Could you check a few things on this model? Use its own coordinates, in mm. A direction names the side the tool comes from. Give positions to 0.01 mm unless a question says otherwise; leave off trailing zeros. Order: outer loops, then holes, each group sorted by start corner. A loop starts at its lowest first (then second) coordinate and runs counter-clockwise, first axis right, second up. Notation, with made-up numbers: M -6.5,9 L 1.5,9 A18 ccw 1.5,26 Z; hole C 86.5,18.25 d3. An arc over 180 degrees is marked long. Use a Markdown table: item, result. Add a question column.
```python
from build123d import *

# Parameters (mm, degrees)
SKETCH_1_W                    = 520
SKETCH_1_H                    = 700
EXTRUDE_1_DEPTH               = 40
SKETCH_2_R                    = 23.1
CUT_EXTRUDE_1_DEPTH           = 873.926113712
CHAMFER_1_SIZE                = 4
M6X1_0_1_D                    = 5
CUT_EXTRUDE_2_DEPTH           = 873.926113712
HOLE_WIZARD_M10_1_D           = 10.5
HOLE_WIZARD_M10_1_CBORE_D     = 21.48
HOLE_WIZARD_M10_1_CBORE_DEPTH = 6.63
HOLE_WIZARD_M6_1_D            = 5
HOLE_WIZARD_M6_1_DEPTH        = 15
HOLE_WIZARD_M6_1_TIP          = 1.502151548


with BuildPart() as part:
    # 草图1 → 凸台-拉伸1 (new body)
    with BuildSketch(Plane.XY):
        with Locations((260, 350)):
            Rectangle(SKETCH_1_W, SKETCH_1_H)
    extrude(amount=EXTRUDE_1_DEPTH)

    # 草图2 → 切除-拉伸1 (cut, through all)
    with BuildSketch(Plane.XY.offset(40)):
        with Locations((140, 60)):
            Circle(SKETCH_2_R)
        with Locations((440, 60)):
            Circle(SKETCH_2_R)
        with Locations((440, 640)):
            Circle(SKETCH_2_R)
        with Locations((140, 640)):
            Circle(SKETCH_2_R)
    extrude(amount=-CUT_EXTRUDE_1_DEPTH, mode=Mode.SUBTRACT)

    # 倒角1
    chamfer_1_edges = [part.edges().sort_by_distance(p)[0] for p in [
        (520, 350, 40),
        (260, 700, 40),
        (0, 350, 40),
        (260, 700, 0),
        (520, 350, 0),
        (260, 0, 0),
        (0, 350, 0),
        (260, 0, 40),
        (0, 700, 20),
        (520, 700, 20),
        (520, 0, 20),
        (0, 0, 20),
    ]]
    chamfer(chamfer_1_edges, length=CHAMFER_1_SIZE)

    # M6x1.0 螺纹孔1 (through all)
    with Locations(Plane.XY.offset(40)):
        with Locations((25, 507.5), (150, 507.5), (275, 507.5), (275, 192.5), (150, 192.5), (25, 192.5)):
            Hole(M6X1_0_1_D / 2)

    # 草图5 → 切除-拉伸2 (cut, through all)
    with BuildSketch(Plane.XY.offset(40)):
        with BuildLine():
            Line((60, 370), (290, 370))
            ThreePointArc((290, 370), (310, 350), (290, 330))
            Line((290, 330), (60, 330))
            ThreePointArc((60, 330), (40, 350), (60, 370))
        make_face()
    extrude(amount=-CUT_EXTRUDE_2_DEPTH, mode=Mode.SUBTRACT)

    # M10 六角头螺钉的柱形沉头孔1 (through all)
    with Locations(Plane.XY.offset(40)):
        with Locations((15, 670), (15, 450), (15, 250), (15, 30), (505, 30), (505, 250), (505, 450), (505, 667.622862113)):
            CounterBoreHole(HOLE_WIZARD_M10_1_D / 2, HOLE_WIZARD_M10_1_CBORE_D / 2, HOLE_WIZARD_M10_1_CBORE_DEPTH)

    # M6 螺纹孔1
    with Locations(Plane(origin=(0, 0, 0), x_dir=(-1, 0, 0), z_dir=(0, -1, 0))):
        with Locations((-260, -20)):
            Hole(HOLE_WIZARD_M6_1_D / 2, depth=HOLE_WIZARD_M6_1_DEPTH)
            with Locations((0, 0, -(HOLE_WIZARD_M6_1_DEPTH + HOLE_WIZARD_M6_1_TIP / 2))):  # 118° drill point
                Cone(0, HOLE_WIZARD_M6_1_D / 2, HOLE_WIZARD_M6_1_TIP, mode=Mode.SUBTRACT)


solid = part.part
```
1) For faces 3 (the face through (520, 345, 20)), 4 (the face through (173, 370, 20)), 5 (the face through (12, 445, 33.37)), which set-ups out of +Z, -Z, +X, -X, +Y, -Y let a thin tool reach every point of the face, with its end or its side?
2) Suppose I cut it at A-A on y = 60. Please give me the cut outline in (x, z), and give its area (3 significant figures).
3) Suppose I cut it at D-D on y = 341. Please give me the cut outline in (x, z).
4) We'd pull the mould along Y, two halves only. Please class faces 1 (the face through (177, 330, 20)), 2 (the face through (313, 355, 40)): pulls with the +Y half, pulls with the -Y half, needs draft (parallel to the pull), parting line crosses it, or undercut.
5) Suppose I cut it at B-B on x = 140. Please give me the cut outline in (y, z), and give its area (3 significant figures).
6) Please list where these lines run through material, in increasing order: line 1 (X direction, y = 507, z = 17); line 2 (Y direction, x = 15, z = 21); line 3 (Y direction, x = 275, z = 30.5). Write a range as from..to.
7) For pin 1 (6.5 mm diameter, centred on x = 10, y = 673, fed in from +Z), with a flat end and sliding along its axis, tell me the tip position at first contact or that it passes through.
8) Suppose I cut it at C-C on x = 207.5. Please give me the cut outline in (y, z), and give its area (3 significant figures).
Values found:
| question | item | result |
|---|---|---|
| 1 | face 3 | +Z, -Z, +X, +Y, -Y |
| 1 | face 4 | +Z, -Z |
| 1 | face 5 | +Z |
| 2 | outline | M 0,4 L 4,0 L 116.9,0 L 116.9,40 L 4,40 L 0,36 Z; M 163.1,0 L 416.9,0 L 416.9,40 L 163.1,40 Z; M 463.1,0 L 516,0 L 520,4 L 520,36 L 516,40 L 463.1,40 Z |
| 2 | area | 17,100 mm^2 |
| 3 | outline | M 0,4 L 4,0 L 42.14,0 L 42.14,40 L 4,40 L 0,36 Z; M 307.86,0 L 516,0 L 520,4 L 520,36 L 516,40 L 307.86,40 Z |
| 4 | face 1 | undercut |
| 4 | face 2 | needs draft |
| 5 | outline | M 0,4 L 4,0 L 36.9,0 L 36.9,40 L 4,40 L 0,36 Z; M 83.1,0 L 330,0 L 330,40 L 83.1,40 Z; M 370,0 L 616.9,0 L 616.9,40 L 370,40 Z; M 663.1,0 L 696,0 L 700,4 L 700,36 L 696,40 L 663.1,40 Z |
| 5 | area | 22,700 mm^2 |
| 6 | line 1 | x = 0..22.55, 27.45..147.55, 152.45..272.55, 277.45..520 |
| 6 | line 2 | y = 0..24.75, 35.25..244.75, 255.25..444.75, 455.25..664.75, 675.25..700 |
| 6 | line 3 | y = 0..190, 195..330, 370..505, 510..700 |
| 7 | pin 1 | stops at z = 33.37 |
| 8 | outline | M 0,4 L 4,0 L 330,0 L 330,40 L 4,40 L 0,36 Z; M 370,0 L 696,0 L 700,4 L 700,36 L 696,40 L 370,40 Z |
| 8 | area | 26,400 mm^2 |
